Check sheet for the modelled part. Datum: model origin and axes. Units: mm. Give positions to 0.01 mm unless a question says otherwise; leave off trailing zeros. Order: outer loops, then holes, each group sorted by start corner. A loop starts at its lowest first (then second) coordinate and runs counter-clockwise, first axis right, second up.
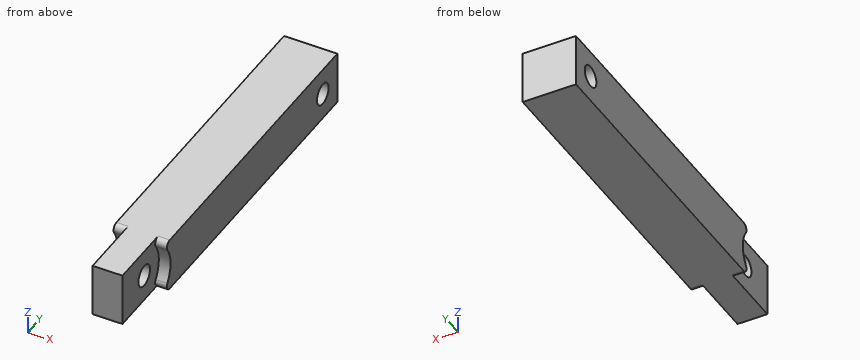
```python
from build123d import *

# Parameters (mm, degrees)
SKETCH1_W               = 50
SKETCH1_H               = 50
BOSS_EXTRUDE1_DEPTH     = 300
SKETCH2_W               = 28
SKETCH2_H               = 50
BOSS_EXTRUDE2_DEPTH     = 48.9
CUT_EXTRUDE4_DEPTH      = 309.220700148
CUT_EXTRUDE4_DEPTH_BACK = 11
CUT_EXTRUDE7_DEPTH      = 11
SKETCH12_R              = 10
CUT_EXTRUDE8_DEPTH      = 307.628439646
FILLET2_R               = 5
FILLET3_R               = 5
SKETCH13_R              = 10
CUT_EXTRUDE9_DEPTH      = 309.220700148


with BuildPart() as part:
    # Sketch1 → Boss-Extrude1 (new body)
    with BuildSketch(Plane(origin=(0, 0, 0), x_dir=(1, 0, 0), z_dir=(0, 1, 0))):
        with Locations((-25, 25)):
            Rectangle(SKETCH1_W, SKETCH1_H)
    extrude(amount=BOSS_EXTRUDE1_DEPTH)

    # Sketch2 → Boss-Extrude2 (add)
    with BuildSketch(Plane.XZ):
        with Locations((-25, -25)):
            Rectangle(SKETCH2_W, SKETCH2_H)
    extrude(amount=BOSS_EXTRUDE2_DEPTH)

    # Sketch5 → Cut-Extrude4 (cut, two sides: drawn at the far end of the back side and taken through both)
    with BuildSketch(Plane(origin=(0, 0, 0), x_dir=(0, 0, -1), z_dir=(1, 0, 0)).offset(-CUT_EXTRUDE4_DEPTH_BACK)):
        with BuildLine():
            Line((50, 0), (0, 0))
            ThreePointArc((0, 0), (25, 13.416876048), (50, 0))
        make_face()
    extrude(amount=CUT_EXTRUDE4_DEPTH + CUT_EXTRUDE4_DEPTH_BACK, mode=Mode.SUBTRACT)

    # Sketch6 → Cut-Extrude7 (cut)
    with BuildSketch(Plane.ZY.offset(50)):
        with BuildLine():
            Line((-50, 0), (0, 0))
            ThreePointArc((0, 0), (-25, 13.416876048), (-50, 0))
        make_face()
    extrude(amount=-CUT_EXTRUDE7_DEPTH, mode=Mode.SUBTRACT)

    # Sketch12 → Cut-Extrude8 (cut, through all)
    with BuildSketch(Plane.ZY.offset(39)):
        with Locations((-25, -11.583123952)):
            Circle(SKETCH12_R)
    extrude(amount=-CUT_EXTRUDE8_DEPTH, mode=Mode.SUBTRACT)

    # Fillet2
    fillet2_edges = [part.edges().sort_by_distance(p)[0] for p in [
        (-44.5, 0, -50),
        (-44.5, 0, 0),
    ]]
    fillet(fillet2_edges, radius=FILLET2_R)

    # Fillet3
    fillet3_edges = [part.edges().sort_by_distance(p)[0] for p in [
        (-5.5, 0, 0),
        (-5.5, 0, -50),
    ]]
    fillet(fillet3_edges, radius=FILLET3_R)

    # Sketch13 → Cut-Extrude9 (cut, through all)
    with BuildSketch(Plane(origin=(0, 0, 0), x_dir=(0, 0, -1), z_dir=(1, 0, 0))):
        with Locations((25, 275)):
            Circle(SKETCH13_R)
    extrude(amount=-CUT_EXTRUDE9_DEPTH, mode=Mode.SUBTRACT)


solid = part.part
```
(1) Go/stop test with flat-tipped pins: P1, Ø1, axis at x = -10, z = -15.5, coming from the -Y side; P2, Ø18, axis at y = 275, z = -25, coming from the -X side; P3, Ø12, axis at y = 226, z = -40, coming from the +X side. Record where each tip stops, or that it passes through.
(2) Sectioned sample at C-C (x = -4.5). Enter the section's corners in (y, z).
(3) Sectioned sample at A-A (y = 275). Enter the section's corners in (x, z).
(4) Thickness scan on L1, parallel to Y at x = -30, z = -25; L2, parallel to Y at x = -37.5, z = -23.5; L3, parallel to Y at x = -10.5, z = -25. Record the ranges inside material, lowest first.
(5) Sectioned sample at B-B (z = -25). Enter the section's corners in (x, y), plus the area to 3 significant figures.
(6) Sectioned sample at D-D (z = -4.5). Enter the section's corners in (x, y).
Values follow:
1. P1: stops at y = 11.7
1. P2: passes through
1. P3: stops at x = 0
2. outline: (8.04, -42.14) arc R5 ccw to (12.14, -50) - (300, -50) - (300, 0) - (12.14, 0) arc R5 ccw to (8.04, -7.86) arc R30 cw to start; hole circle Ø20 at (275, -25)
3. outline: (-50, -50) - (0, -50) - (0, -35) - (-50, -35) - close; (-50, -15) - (0, -15) - (0, 0) - (-50, 0) - close
4. L1: y = -48.9 to -21.58, -1.58 to 265, 285 to 300
4. L2: y = -48.9 to -21.47, -1.7 to 265.11, 284.89 to 300
4. L3: y = 13.42 to 265, 285 to 300
5. outline: (-50, 13.42) - (-39, 13.42) - (-39, -1.58) - (-11, -1.58) - (-11, 13.42) - (0, 13.42) - (0, 265) - (-50, 265) - close; (-50, 285) - (0, 285) - (0, 300) - (-50, 300) - close; (-39, -48.9) - (-11, -48.9) - (-11, -21.58) - (-39, -21.58) - close
5. area: 14,500 mm2
6. outline: (-50, 7.16) - (-39, 7.16) - (-39, -48.9) - (-11, -48.9) - (-11, 7.16) - (0, 7.16) - (0, 300) - (-50, 300) - close
